Check sheet for the drawn part. Datum: minimum x, y, z corner. Units: mm. Round coordinates to 2 decimals unless told otherwise and drop trailing zeros. Loops run counter-clockwise (first coordinate to the right, second up) from the corner with the lowest first, then second, coordinate; pieces in that order, holes last.
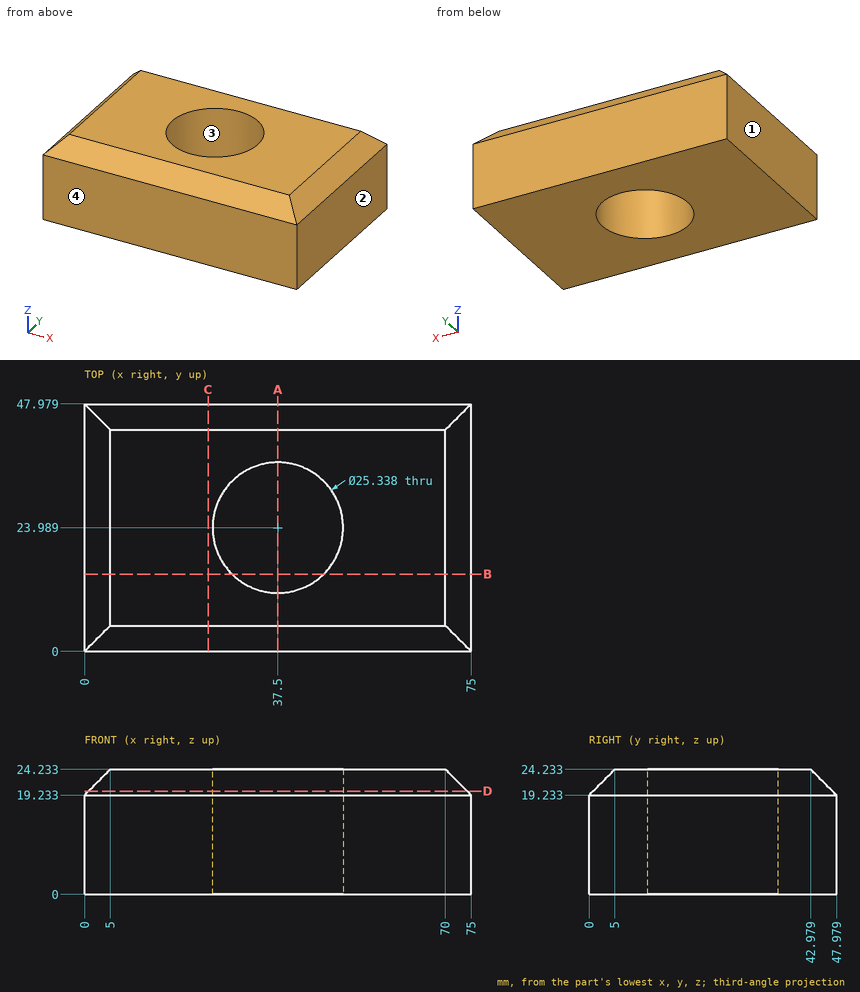
1. Section check A-A (x = 37.5). Enter the section's corners in (y, z).
2. Section check C-C (x = 24). Enter the section's corners in (y, z), then the cut area to 3 significant figures.
3. Section check B-B (y = 15). Enter the section's corners in (x, z).
4. Section check D-D (z = 20). Enter the section's corners in (x, y).
5. Scan lines: L1, parallel to Y at x = 37.5, z = 5.5; L2, parallel to X at y = 24, z = 17; L3, parallel to X at y = 33.5, z = 22 (1 decimal). Record each from-to range of solid material in increasing order.
6. Release check for a two-part mould opening along X. For the marked faces 1, 2, 3 and 4 record: released by +X, released by -X, zero draft, split by the parting line, or undercut.
Taken from the geometry:
1. outline: (0, 0) - (11.32, 0) - (11.32, 24.23) - (5, 24.23) - (0, 19.23) - close; (36.66, 0) - (47.98, 0) - (47.98, 19.23) - (42.98, 24.23) - (36.66, 24.23) - close
2. outline: (0, 0) - (47.98, 0) - (47.98, 19.23) - (42.98, 24.23) - (5, 24.23) - (0, 19.23) - close
2. area: 1,140 mm2
3. outline: (0, 0) - (28.57, 0) - (28.57, 24.23) - (5, 24.23) - (0, 19.23) - close; (46.43, 0) - (75, 0) - (75, 19.23) - (70, 24.23) - (46.43, 24.23) - close
4. outline: (0.77, 0.77) - (74.23, 0.77) - (74.23, 47.21) - (0.77, 47.21) - close; hole circle Ø25.34 at (37.5, 23.99)
5. L1: y = 0 to 11.32, 36.66 to 47.98
5. L2: x = 0 to 24.83, 50.17 to 75
5. L3: x = 2.8 to 29.1, 45.9 to 72.2
6. face 1: released by -X
6. face 2: released by +X
6. face 3: undercut
6. face 4: zero draft
